```python
from build123d import *

# Parameters (mm, degrees)
CROQUIS2_R              = 4.25
SALIENTE_EXTRUIR1_DEPTH = 5
CORTAR_EXTRUIR1_REACH   = 75.527
CROQUIS3_R              = 2.25


with BuildPart() as part:
    # Croquis1 → Revolución1 (revolve)
    with BuildSketch(Plane.XY, mode=Mode.PRIVATE) as revoluci_n1_sk:
        Polygon((32.5, 0), (-32.5, 0), (-32.5, 4), (-17, 4), (-17, 6), (-5, 6), (-5, 20), (5, 20), (5, 6), (17, 6), (17, 4), (32.5, 4), align=None)
    revolve(revoluci_n1_sk.sketch.rotate(Axis((32.5, 0, 0), (-1, 0, 0)), 90), axis=Axis((32.5, 0, 0), (-1, 0, 0)))

    # Croquis2 → Saliente-Extruir1 (add, symmetric)
    with BuildSketch(Plane(origin=(0, 0, 0), x_dir=(0, 0, -1), z_dir=(1, 0, 0))):
        with BuildLine():
            Line((-52, 9.797958971), (-4, 19.595917942))
            ThreePointArc((-4, 19.595917942), (20, 0), (-4, -19.595917942))
            Line((-4, -19.595917942), (-52, -9.797958971))
            ThreePointArc((-52, -9.797958971), (-60, 0), (-52, 9.797958971))
        make_face()
        with Locations((-50, 0)):
            Circle(CROQUIS2_R, mode=Mode.SUBTRACT)
    extrude(amount=SALIENTE_EXTRUIR1_DEPTH, both=True)

    # Croquis3 → Cortar-Extruir1 (cut, up to next)
    with BuildSketch(Plane(origin=(5, 0, 0), x_dir=(0, 0, -1), z_dir=(1, 0, 0)), mode=Mode.PRIVATE) as cortar_extruir1_sk1:
        with Locations((0, 13.75)):
            Circle(CROQUIS3_R)
    cortar_extruir1_tool1 = extrude(cortar_extruir1_sk1.sketch, amount=-CORTAR_EXTRUIR1_REACH, mode=Mode.PRIVATE) & part.part
    # Croquis3 → Cortar-Extruir1 (cut, up to next)
    with BuildSketch(Plane(origin=(5, 0, 0), x_dir=(0, 0, -1), z_dir=(1, 0, 0)), mode=Mode.PRIVATE) as cortar_extruir1_sk2:
        with Locations((11.907849302, 6.875)):
            Circle(CROQUIS3_R)
    cortar_extruir1_tool2 = extrude(cortar_extruir1_sk2.sketch, amount=-CORTAR_EXTRUIR1_REACH, mode=Mode.PRIVATE) & part.part
    # Croquis3 → Cortar-Extruir1 (cut, up to next)
    with BuildSketch(Plane(origin=(5, 0, 0), x_dir=(0, 0, -1), z_dir=(1, 0, 0)), mode=Mode.PRIVATE) as cortar_extruir1_sk3:
        with Locations((11.907849302, -6.875)):
            Circle(CROQUIS3_R)
    cortar_extruir1_tool3 = extrude(cortar_extruir1_sk3.sketch, amount=-CORTAR_EXTRUIR1_REACH, mode=Mode.PRIVATE) & part.part
    # Croquis3 → Cortar-Extruir1 (cut, up to next)
    with BuildSketch(Plane(origin=(5, 0, 0), x_dir=(0, 0, -1), z_dir=(1, 0, 0)), mode=Mode.PRIVATE) as cortar_extruir1_sk4:
        with Locations((0, -13.75)):
            Circle(CROQUIS3_R)
    cortar_extruir1_tool4 = extrude(cortar_extruir1_sk4.sketch, amount=-CORTAR_EXTRUIR1_REACH, mode=Mode.PRIVATE) & part.part
    # Croquis3 → Cortar-Extruir1 (cut, up to next)
    with BuildSketch(Plane(origin=(5, 0, 0), x_dir=(0, 0, -1), z_dir=(1, 0, 0)), mode=Mode.PRIVATE) as cortar_extruir1_sk5:
        with Locations((-11.907849302, -6.875)):
            Circle(CROQUIS3_R)
    cortar_extruir1_tool5 = extrude(cortar_extruir1_sk5.sketch, amount=-CORTAR_EXTRUIR1_REACH, mode=Mode.PRIVATE) & part.part
    # Croquis3 → Cortar-Extruir1 (cut, up to next)
    with BuildSketch(Plane(origin=(5, 0, 0), x_dir=(0, 0, -1), z_dir=(1, 0, 0)), mode=Mode.PRIVATE) as cortar_extruir1_sk6:
        with Locations((-11.907849302, 6.875)):
            Circle(CROQUIS3_R)
    cortar_extruir1_tool6 = extrude(cortar_extruir1_sk6.sketch, amount=-CORTAR_EXTRUIR1_REACH, mode=Mode.PRIVATE) & part.part
    add(cortar_extruir1_tool1.solids().sort_by_distance((5, 13.75, 0))[0], mode=Mode.SUBTRACT)
    add(cortar_extruir1_tool2.solids().sort_by_distance((5, 6.875, -11.907849))[0], mode=Mode.SUBTRACT)
    add(cortar_extruir1_tool3.solids().sort_by_distance((5, -6.875, -11.907849))[0], mode=Mode.SUBTRACT)
    add(cortar_extruir1_tool4.solids().sort_by_distance((5, -13.75, 0))[0], mode=Mode.SUBTRACT)
    add(cortar_extruir1_tool5.solids().sort_by_distance((5, -6.875, 11.907849))[0], mode=Mode.SUBTRACT)
    add(cortar_extruir1_tool6.solids().sort_by_distance((5, 6.875, 11.907849))[0], mode=Mode.SUBTRACT)


solid = part.part
```
Input: part model. Units: mm. Frame: model coordinates. A direction names the side the tool comes from. Give positions to 0.01 mm unless a question says otherwise; leave off trailing zeros. Order: outer loops, then holes, each group sorted by start corner. A loop starts at its lowest first (then second) coordinate and runs counter-clockwise, first axis right, second up. Notation, with made-up numbers: M -7.75,30.5 L 10.25,30.5 A31 ccw 10.25,55.5 Z; hole C 62.5,19.5 d4. An arc over 180 degrees is marked long. Return JSON: item names as keys, results as strings.
Item 1: Cut plane B-B (y = 0). Return loops of the section in (x, z), then the cut area to 3 significant figures.
Solutions:
{"outline": "M -32.5,-4 L -17,-4 L -17,-6 L -5,-6 L -5,-20 L 5,-20 L 5,-6 L 17,-6 L 17,-4 L 32.5,-4 L 32.5,4 L 17,4 L 17,6 L 5,6 L 5,45.75 L -5,45.75 L -5,6 L -17,6 L -17,4 L -32.5,4 Z; M -5,54.25 L 5,54.25 L 5,60 L -5,60 Z", "area": "1,250 mm^2"}
Item 2: Cut plane C-C (x = -2). Return loops of the section in (y, z) (3 decimals).
Solutions:
{"outline": "M -19.596,4 A20 ccw long 19.596,4 L 9.798,52 A10 ccw -9.798,52 Z; hole C -13.75,0 d4.5; hole C -6.875,-11.908 d4.5; hole C -6.875,11.908 d4.5; hole C 0,50 d8.5; hole C 6.875,-11.908 d4.5; hole C 6.875,11.908 d4.5; hole C 13.75,0 d4.5"}
Item 3: Pull-direction query (Y, two-part tool) for faces 1 (the flat face through (0.07, 14.628, 28.336)), 2 (the cylindrical face through (0, -16, 0)), 3 (the cylindrical face through (0, 0, -20)); classes: +Y half, -Y half, draft (parallel to the pull), parting line (faces both ways), or undercut.
Solutions:
{"face 1": "+Y half", "face 2": "undercut", "face 3": "parting line"}
Item 4: Cut plane D-D (x = 6.5). Return loops of the section in (y, z).
Solutions:
{"outline": "C 0,0 d12"}
Item 5: Cut plane A-A (z = 0). Return loops of the section in (x, y), then the cut area to 3 significant figures.
Solutions:
{"outline": "M -32.5,-4 L -17,-4 L -17,-6 L -5,-6 L -5,-11.5 L 5,-11.5 L 5,-6 L 17,-6 L 17,-4 L 32.5,-4 L 32.5,4 L 17,4 L 17,6 L 5,6 L 5,11.5 L -5,11.5 L -5,6 L -17,6 L -17,4 L -32.5,4 Z; M -5,-20 L 5,-20 L 5,-16 L -5,-16 Z; M -5,16 L 5,16 L 5,20 L -5,20 Z", "area": "846 mm^2"}
Item 6: First-contact query: P1, Ø1.5, axis at y = 15.5, z = 31.5, coming from the -X side; P2, Ø4, axis at y = -12, z = -10, coming from the +X side; P3, Ø8, axis at x = -18, y = 3, coming from the -Z side; P4, Ø6, axis at x = -0.5, y = 10.5, coming from the +Z side. Flat tips, straight axial feed; report the tip coordinate or a pass-through.
Solutions:
{"P1": "through", "P2": "x = 5", "P3": "z = -6", "P4": "z = 56.61"}
Item 7: Access query for faces 4 (the cylindrical face through (11.084, -1.802, -5.723)), 5 (the flat face through (-17, 3.92, -1.42)), 6 (the cylindrical face through (0.07, -6.2, 9.76)). Directions: +Z, -Z, +X, -X, +Y, -Y. A direction counts if a zero-diameter tool reaches every point of the face in a straight line with its end or side. Return the directions, or none.
Solutions:
{"face 4": "+X", "face 5": "-X", "face 6": "+X, -X"}
Item 8: Ray query, probe 1 along Y at (x, z) = (2, 0); probe 2 along X at (y, z) = (9, -13); probe 3 along Z at (x, y) = (-3, 3). Return the intervals inside material, ascending.
Solutions:
{"probe 1": "-20 to -16, -11.5 to 11.5, 16 to 20", "probe 2": "-5 to 5", "probe 3": "-19.77 to 46.99, 53.01 to 59.54"}
